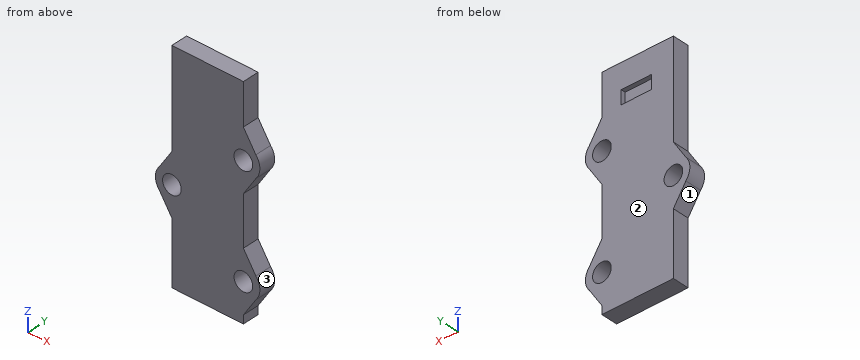
```python
from build123d import *

# Parameters (mm, degrees)
BOX031_W               = 5.5
BOX031_H               = 10
BOX031_DEPTH           = 2.5
CYLINDER059_R          = 1.7
CYLINDER059_DEPTH      = 30
CYLINDER059_ROLL_ANGLE = 90
CYLINDER060_R          = 1.7
CYLINDER060_DEPTH      = 30
CYLINDER060_ROLL_ANGLE = 90
CYLINDER058_R          = 1.7
CYLINDER058_DEPTH      = 30
CYLINDER058_ROLL_ANGLE = 90
CYLINDER056_R          = 3
CYLINDER056_DEPTH      = 3
CYLINDER056_ROLL_ANGLE = 90
CYLINDER057_R          = 3
CYLINDER057_DEPTH      = 3
CYLINDER057_ROLL_ANGLE = 90
CYLINDER055_R          = 3
CYLINDER055_DEPTH      = 3
CYLINDER055_ROLL_ANGLE = 90
BOX029_W               = 13
BOX029_H               = 3
BOX029_DEPTH           = 40
CHAMFER007_SIZE        = 2.5


with BuildPart() as m3_nut_hole001:
    # Box031 → Box031 (new body)
    with BuildSketch(Plane(origin=(59, 11.7, 74), x_dir=(1, 0, 0), z_dir=(0, 0, 1))):
        with Locations((2.75, 5)):
            Rectangle(BOX031_W, BOX031_H)
    extrude(amount=BOX031_DEPTH)


with BuildPart() as cylinder098:
    # Cylinder059 → Cylinder059 (new body)
    with BuildSketch(Plane.XY):
        Circle(CYLINDER059_R)
    extrude(amount=CYLINDER059_DEPTH)


with BuildPart() as cylinder098_1:
    # Cylinder059 roll: moved
    add(cylinder098.part.rotate(Axis((0, 0, 0), (1, 0, 0)), CYLINDER059_ROLL_ANGLE))


with BuildPart() as cylinder098_2:
    # Cylinder059 placement: moved
    add(cylinder098_1.part.moved(Location((68, 26, 48))))


with BuildPart() as cylinder059:
    # Cylinder060 → Cylinder060 (new body)
    with BuildSketch(Plane.XY):
        Circle(CYLINDER060_R)
    extrude(amount=CYLINDER060_DEPTH)


with BuildPart() as cylinder059_1:
    # Cylinder060 roll: moved
    add(cylinder059.part.rotate(Axis((0, 0, 0), (1, 0, 0)), CYLINDER060_ROLL_ANGLE))


with BuildPart() as cylinder059_2:
    # Cylinder060 placement: moved
    add(cylinder059_1.part.moved(Location((68, 27, 68))))


with BuildPart() as fusion032:
    # Cylinder058 → Cylinder058 (new body)
    with BuildSketch(Plane.XY):
        Circle(CYLINDER058_R)
    extrude(amount=CYLINDER058_DEPTH)


with BuildPart() as fusion032_1:
    # Cylinder058 roll: moved
    add(fusion032.part.rotate(Axis((0, 0, 0), (1, 0, 0)), CYLINDER058_ROLL_ANGLE))


with BuildPart() as fusion032_2:
    # Cylinder058 placement: moved
    add(fusion032_1.part.moved(Location((55, 26, 58))))

    # Fusion032: union Cylinder098, Cylinder059
    add(cylinder098_2.part)
    add(cylinder059_2.part)


with BuildPart() as cylinder095:
    # Cylinder056 → Cylinder056 (new body)
    with BuildSketch(Plane.XY):
        Circle(CYLINDER056_R)
    extrude(amount=CYLINDER056_DEPTH)


with BuildPart() as cylinder095_1:
    # Cylinder056 roll: moved
    add(cylinder095.part.rotate(Axis((0, 0, 0), (1, 0, 0)), CYLINDER056_ROLL_ANGLE))


with BuildPart() as cylinder095_2:
    # Cylinder056 placement: moved
    add(cylinder095_1.part.moved(Location((68, 12.5, 68))))


with BuildPart() as cylinder096:
    # Cylinder057 → Cylinder057 (new body)
    with BuildSketch(Plane.XY):
        Circle(CYLINDER057_R)
    extrude(amount=CYLINDER057_DEPTH)


with BuildPart() as cylinder096_1:
    # Cylinder057 roll: moved
    add(cylinder096.part.rotate(Axis((0, 0, 0), (1, 0, 0)), CYLINDER057_ROLL_ANGLE))


with BuildPart() as cylinder096_2:
    # Cylinder057 placement: moved
    add(cylinder096_1.part.moved(Location((68, 12.5, 48))))


with BuildPart() as trolley_hubs_b:
    # Cylinder055 → Cylinder055 (new body)
    with BuildSketch(Plane.XY):
        Circle(CYLINDER055_R)
    extrude(amount=CYLINDER055_DEPTH)


with BuildPart() as trolley_hubs_b_1:
    # Cylinder055 roll: moved
    add(trolley_hubs_b.part.rotate(Axis((0, 0, 0), (1, 0, 0)), CYLINDER055_ROLL_ANGLE))


with BuildPart() as trolley_hubs_b_2:
    # Cylinder055 placement: moved
    add(trolley_hubs_b_1.part.moved(Location((55, 12.5, 58))))

    # Fusion050: union Cylinder095, Cylinder096
    add(cylinder095_2.part)
    add(cylinder096_2.part)


with BuildPart() as trolley_plate:
    # Box029 → Box029 (new body)
    with BuildSketch(Plane(origin=(55, 9.5, 41), x_dir=(1, 0, 0), z_dir=(0, 0, 1))):
        with Locations((6.5, 1.5)):
            Rectangle(BOX029_W, BOX029_H)
    extrude(amount=BOX029_DEPTH)

    # Fusion051: union trolley-hubs-b
    add(trolley_hubs_b_2.part)

    # Chamfer007
    chamfer007_edges = [trolley_plate.edges().sort_by_distance(p)[0] for p in [
        (55, 11, 55),
        (68, 11, 45),
        (55, 11, 61),
        (68, 11, 65),
        (68, 11, 51),
        (68, 11, 71),
    ]]
    chamfer(chamfer007_edges, length=CHAMFER007_SIZE)

    # Cut039: cut Fusion032
    add(fusion032_2.part, mode=Mode.SUBTRACT)

    # Cut040: cut M3-nut-hole001
    add(m3_nut_hole001.part, mode=Mode.SUBTRACT)


solid = trolley_plate.part
```
Part model, mm, in its own coordinate system. Face numbers are marked on the shaded views. Give positions to 0.01 mm unless a question says otherwise; leave off trailing zeros. Loops run counter-clockwise (first coordinate to the right, second up) from the corner with the lowest first, then second, coordinate; pieces in that order, holes last. Notation, with made-up numbers: M 13,-22 L 54,-22 A20 cw 54,13 Z; hole C 58,88 d10. An arc over 180 degrees is marked long. Return JSON: item names as keys, results as strings.
1) Saw through at A-A, the plane z = 58. List the corners of the cut face in (x, y).
Calculated:
{"outline": "M 52,9.5 L 53.3,9.5 L 53.3,12.5 L 52,12.5 Z; M 56.7,9.5 L 68,9.5 L 68,12.5 L 56.7,12.5 Z"}
2) Pull direction Z, two halves, no side cores. Call the marked faces 1, 2 and 3: released by +Z, released by -Z, zero draft, split by the parting line, or undercut.
Calculated:
{"face 1": "released by -Z", "face 2": "zero draft", "face 3": "undercut"}
3) Saw through at C-C, the plane y = 10.35. Count the separate pieces of the cut face and the enclosed holes in it, then the cut area to 3 significant figures.
Calculated:
{"separate pieces": "1", "enclosed holes": "3", "area": "549 mm2"}
4) Flat gauge pins, fed straight in: pin 1 Ø0.6 at (y, z) = (12, 75.5) entering from -X; pin 2 Ø2 at (x, z) = (55, 58) entering from -Y; pin 3 Ø4 at (x, z) = (68.5, 53.5) entering from +Y; pin 4 Ø1.5 at (y, z) = (11.5, 56) entering from +X. Where does each tip first touch, or does it go through?
Calculated:
{"pin 1": "stops at x = 55", "pin 2": "passes through", "pin 3": "stops at y = 12.5", "pin 4": "stops at x = 68"}
5) Saw through at B-B, the plane x = 54.5. List the corners of the cut face in (y, z).
Calculated:
{"outline": "M 9.5,53.28 L 12.5,53.28 L 12.5,56.38 L 9.5,56.38 Z; M 9.5,59.62 L 12.5,59.62 L 12.5,62.72 L 9.5,62.72 Z"}
6) Drill centre lines: line 1 (Z direction, x = 60, y = 11.9); line 2 (Z direction, x = 68.5, y = 11.4); line 3 (X direction, y = 10.7, z = 48). Where is each one in solid material? Low to high.
Calculated:
{"line 1": "z = 41 to 74, 76.5 to 81", "line 2": "z = 43.28 to 46.38, 49.62 to 52.72, 63.28 to 66.38, 69.62 to 72.72", "line 3": "x = 55 to 66.3, 69.7 to 71"}
